from build123d import *

# Parameters (mm, degrees)
SKETCH1_W           = 40.15
SKETCH1_H           = 20.15
BOSS_EXTRUDE1_DEPTH = 20.13
SKETCH2_R           = 6.2
BOSS_EXTRUDE2_DEPTH = 1.3
SKETCH3_R           = 3
BOSS_EXTRUDE3_DEPTH = 4
SKETCH7_R           = 2.95
BOSS_EXTRUDE4_DEPTH = 4


with BuildPart() as part:
    # Sketch1 → Boss-Extrude1 (new, symmetric)
    with BuildSketch(Plane(origin=(0, 0, 0), x_dir=(0, 1, 0), z_dir=(0, 0, 1))):
        Rectangle(SKETCH1_W, SKETCH1_H)
    extrude(amount=BOSS_EXTRUDE1_DEPTH, both=True)

    # Sketch2 → Boss-Extrude2 (add)
    with BuildSketch(Plane.XY.offset(20.13)):
        with Locations((0, -10.205)):
            Circle(SKETCH2_R)
    boss_extrude2 = extrude(amount=BOSS_EXTRUDE2_DEPTH)

    # Mirror1: Boss-Extrude2 across plane
    add(boss_extrude2.mirror(Plane.XY))

    # Sketch3 → Boss-Extrude3 (add)
    with BuildSketch(Plane(origin=(0, 0, -21.43), x_dir=(1, 0, 0), z_dir=(0, 0, -1))):
        with Locations(Location((0, 10.205, 0), (0, 0, 180))):
            Circle(SKETCH3_R)
    extrude(amount=BOSS_EXTRUDE3_DEPTH)

    # Sketch7 → Boss-Extrude4 (add)
    with BuildSketch(Plane.XY.offset(21.43)):
        with Locations((0, -10.205)):
            Circle(SKETCH7_R)
    extrude(amount=BOSS_EXTRUDE4_DEPTH)


solid = part.part
Input: part model. Units: mm. Frame: model coordinates. A direction names the side the tool comes from. Round coordinates to 2 decimals unless told otherwise and drop trailing zeros. Order: outer loops, then holes, each group sorted by start corner. A loop starts at its lowest first (then second) coordinate and runs counter-clockwise, first axis right, second up. Notation, with made-up numbers: (51.5, -33) - (92.5, -33) arc R26 cw to (92.5, -11) - close; hole circle Ø6 at (69, -39.5). An arc over 180 degrees is marked (long way). Use a Markdown table: item, result.
1. Access query for faces 1 (the face through (-0.81, -4.06, 20.77)), 2 (the face through (3, -9, -21.43)), 3 (the face through (0, -20.075, 0)). Directions: +Z, -Z, +X, -X, +Y, -Y. A direction counts if a zero-diameter tool reaches every point of the face in a straight line with its end or side. Return the directions, or none.
Evaluation:
| item | result |
|---|---|
| face 1 | +Z |
| face 2 | -Z |
| face 3 | +Z, -Z, +X, -X, -Y |
2. Section A-A on x = 0. Return the cut outline in (y, z) (3 decimals).
Evaluation:
| item | result |
|---|---|
| outline | (-20.075, -20.13) - (-16.405, -20.13) - (-16.405, -21.43) - (-13.205, -21.43) - (-13.205, -25.43) - (-7.205, -25.43) - (-7.205, -21.43) - (-4.005, -21.43) - (-4.005, -20.13) - (20.075, -20.13) - (20.075, 20.13) - (-4.005, 20.13) - (-4.005, 21.43) - (-7.255, 21.43) - (-7.255, 25.43) - (-13.155, 25.43) - (-13.155, 21.43) - (-16.405, 21.43) - (-16.405, 20.13) - (-20.075, 20.13) - close |
3. Section B-B on y = -17. Return the cut outline in (x, z) (3 decimals), then the cut area to 3 significant figures.
Evaluation:
| item | result |
|---|---|
| outline | (-10.075, -20.13) - (10.075, -20.13) - (10.075, 20.13) - (-10.075, 20.13) - close |
| area | 811 mm^2 |
4. First-contact query: pin 1 (10 mm diameter, centred on x = -1.5, y = 6, fed in from +Z); pin 2 (6 mm diameter, centred on x = 0.5, y = 12.5, fed in from -Z); pin 3 (4 mm diameter, centred on x = 5, y = -5, fed in from +Z). Flat tips, straight axial feed; report the tip coordinate or a pass-through.
Evaluation:
| item | result |
|---|---|
| pin 1 | z = 20.13 |
| pin 2 | z = -20.13 |
| pin 3 | z = 21.43 |
5. Section D-D on y = -6.5. Return the cut outline in (x, z) (3 decimals).
Evaluation:
| item | result |
|---|---|
| outline | (-10.075, -20.13) - (-4.971, -20.13) - (-4.971, -21.43) - (4.971, -21.43) - (4.971, -20.13) - (10.075, -20.13) - (10.075, 20.13) - (4.971, 20.13) - (4.971, 21.43) - (-4.971, 21.43) - (-4.971, 20.13) - (-10.075, 20.13) - close |
6. Material intervals for probe 1 along Z at (x, y) = (9, 5); probe 2 along Z at (x, y) = (0, -5), sorted ascending.
Evaluation:
| item | result |
|---|---|
| probe 1 | -20.13 to 20.13 |
| probe 2 | -21.43 to 21.43 |
7. Section C-C on x = 5.25. Return the cut outline in (y, z) (3 decimals), then the cut area to 3 significant figures.
Evaluation:
| item | result |
|---|---|
| outline | (-20.075, -20.13) - (-13.503, -20.13) - (-13.503, -21.43) - (-6.907, -21.43) - (-6.907, -20.13) - (20.075, -20.13) - (20.075, 20.13) - (-6.907, 20.13) - (-6.907, 21.43) - (-13.503, 21.43) - (-13.503, 20.13) - (-20.075, 20.13) - close |
| area | 1,630 mm^2 |
